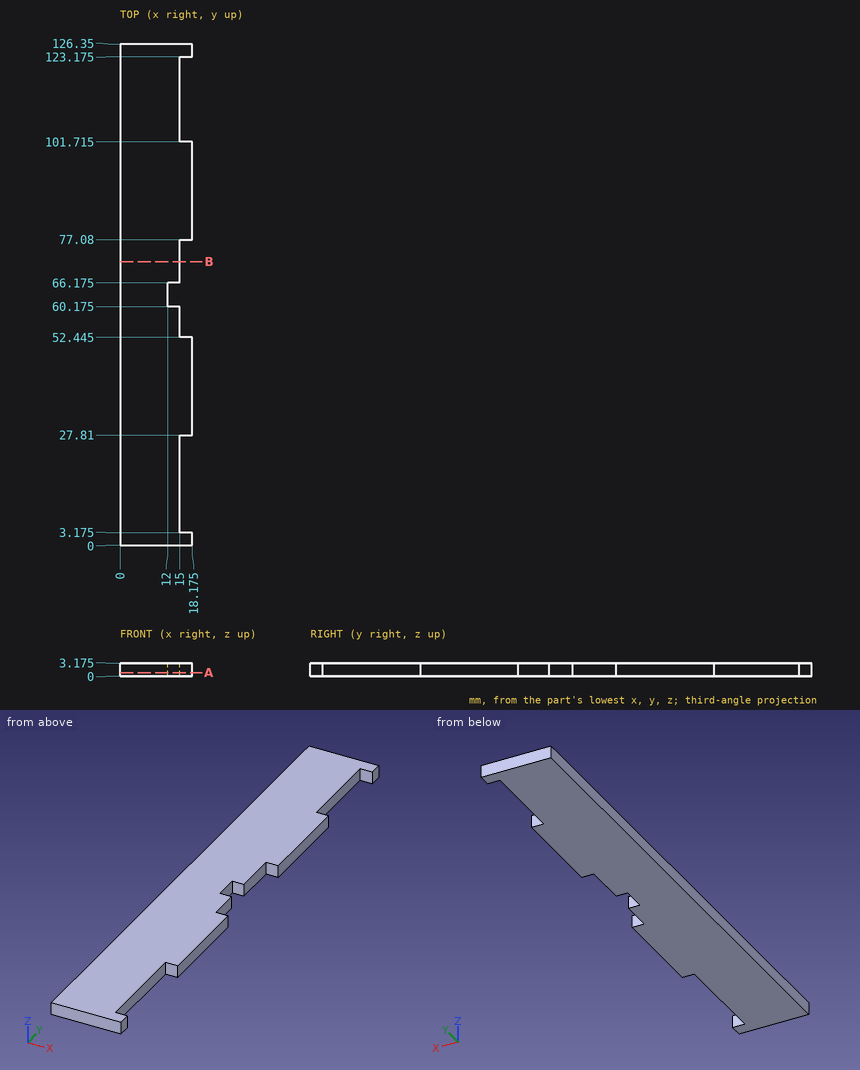
Drawing for the job (mm, zero at the part's lowest x, y, z). Round coordinates to 2 decimals unless told otherwise and drop trailing zeros. Loops run counter-clockwise (first coordinate to the right, second up) from the corner with the lowest first, then second, coordinate; pieces in that order, holes last. Notation, with made-up numbers: (27, -24) -> (63, -24) arc R22 cw to (63, -16) -> close; hole circle Ø6 at (-18, 76.25). An arc over 180 degrees is marked (long way). Answer as CSV lines item,"result". Start each with the question number.
1) Pin check, flat tips, straight feed: P1, Ø1.6, axis at y = 14, z = 1.5, coming from the +X side; P2, Ø5, axis at x = 4.5, y = 111, coming from the -Z side. Stop position of each tip, or through.
2) Probe line 1 along Y through (x, z) = (16, 2.4) (3 decimals); line 2 along Y through (x, z) = (12.5, 1.5) (3 decimals); line 3 along X through (y, z) = (65, 1.95). List the from-to ranges inside material, lowest first.
3) Slice it at A-A (z = 0.85). List the corners of the cut face in (x, y) (3 decimals).
4) Slice it at B-B (y = 71.5). List the corners of the cut face in (x, z) (3 decimals).
Filled in:
1,P1,"stops at x = 15"
1,P2,"stops at z = 0"
2,line 1,"y = 0 to 3.175, 27.81 to 52.445, 77.08 to 101.715, 123.175 to 126.35"
2,line 2,"y = 0 to 60.175, 66.175 to 126.35"
2,line 3,"x = 0 to 12"
3,outline,"(0, 0) -> (18.175, 0) -> (18.175, 3.175) -> (15, 3.175) -> (15, 27.81) -> (18.175, 27.81) -> (18.175, 52.445) -> (15, 52.445) -> (15, 60.175) -> (12, 60.175) -> (12, 66.175) -> (15, 66.175) -> (15, 77.08) -> (18.175, 77.08) -> (18.175, 101.715) -> (15, 101.715) -> (15, 123.175) -> (18.175, 123.175) -> (18.175, 126.35) -> (0, 126.35) -> close"
4,outline,"(0, 0) -> (15, 0) -> (15, 3.175) -> (0, 3.175) -> close"
